```python
from build123d import *

# Parameters (mm, degrees)
BOSS_EXTRUDE1_DEPTH           = 3.175
TAP_DRILL_FOR_8_32_TAP1_D     = 3.4544
TAP_DRILL_FOR_8_32_TAP1_DEPTH = 3.302
TAP_DRILL_FOR_8_32_TAP1_TIP   = 1.037806461
BOSS_EXTRUDE2_DEPTH           = 12.7
F_8_CLEARANCE_HOLE1_D         = 4.9149


with BuildPart() as part:
    # Sketch1 → Boss-Extrude1 (new body)
    with BuildSketch(Plane.XY):
        with BuildLine():
            Line((-9.149583802, 21.93801689), (-26.580783626, -25.95381102))
            Line((-26.580783626, -25.95381102), (20.215712306, -25.95381102))
            Line((20.215712306, -25.95381102), (2.784512482, 21.93801689))
            ThreePointArc((2.784512482, 21.93801689), (-3.18253566, 26.11618898), (-9.149583802, 21.93801689))
        make_face()
    extrude(amount=BOSS_EXTRUDE1_DEPTH)

    # Tap Drill for #8-32 Tap1
    with Locations(Plane(origin=(-3.18253566, 19.76618898, 0), x_dir=(-1, 0, 0), z_dir=(0, 0, -1))):
        with Locations((0, 0)):
            Hole(TAP_DRILL_FOR_8_32_TAP1_D / 2, depth=TAP_DRILL_FOR_8_32_TAP1_DEPTH)
            with Locations((0, 0, -(TAP_DRILL_FOR_8_32_TAP1_DEPTH + TAP_DRILL_FOR_8_32_TAP1_TIP / 2))):  # 118° drill point
                Cone(0, TAP_DRILL_FOR_8_32_TAP1_D / 2, TAP_DRILL_FOR_8_32_TAP1_TIP, mode=Mode.SUBTRACT)

    # Sketch3 → Boss-Extrude2 (add)
    with BuildSketch(Plane(origin=(0, 0, 0), x_dir=(-1, 0, 0), z_dir=(0, 0, -1))):
        Polygon((-19.060106812, -22.77881102), (-20.215712306, -25.95381102), (26.580783626, -25.95381102), (25.425178132, -22.77881102), align=None)
    extrude(amount=BOSS_EXTRUDE2_DEPTH)

    # #8 Clearance Hole1 (through all)
    with Locations(Plane(origin=(-14.303856896, -22.77881102, -6.35), x_dir=(1, 0, 0), z_dir=(0, 1, 0))):
        with Locations((0, 0), (22.242642472, 0)):
            Hole(F_8_CLEARANCE_HOLE1_D / 2)


solid = part.part
```
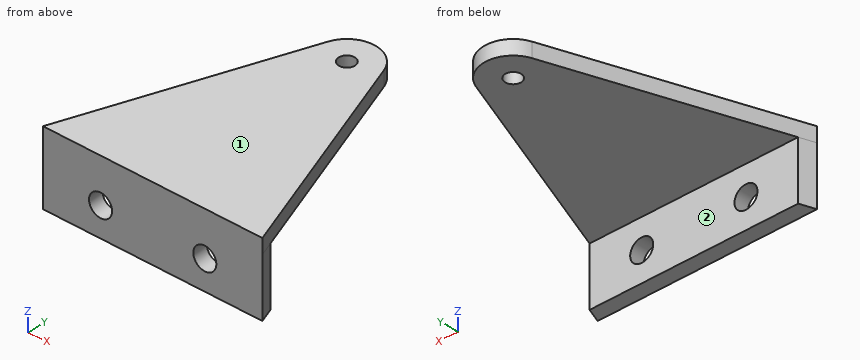
Design review of the part built by this model. Coordinates are the model's own, in mm. Face numbers are marked on the shaded views. A direction names the side the tool comes from. Round coordinates to 2 decimals unless told otherwise and drop trailing zeros. Write each loop counter-clockwise with the first axis right and the second up, starting at its lowest first coordinate (ties: lowest second). Pieces come first, ordered by that corner, then holes.
Item 1: For probe 1 along Z at (x, y) = (-4.5, 10) (3 decimals); probe 2 along Y at (x, z) = (-14, -3.75); probe 3 along X at (y, z) = (-20, 0.5), list the stretches that pass through material, from the lowest coordinate up.
Item 2: We need section B-B on x = 7. Write out the cut boundary in (y, z) (3 decimals).
Item 3: For the marked faces 1 and 2, list the 3-axis set-ups (+Z, -Z, +X, -X, +Y, -Y) from which the entire face can be reached by the end or side of a thin tool; tool diameter is ignored.
Item 4: We need section A-A on z = -6.35. Write out the cut boundary in (x, y), and give its area (3 significant figures).
Item 5: We need section D-D on y = -20.5. Write out the cut boundary in (x, z) (3 decimals).
Item 6: We need section C-C on x = -6. Write out the cut boundary in (y, z) (3 decimals).
Item 7: Clearance check with flat-ended pins moving along their axes: pin 1 Ø1 at (x, z) = (11.5, -4) entering from +Y; pin 2 Ø3 at (x, z) = (7.94, -6.35) entering from +Y; pin 3 Ø22 at (x, y) = (0.5, 9) entering from -Z; pin 4 Ø4 at (y, z) = (14.5, -0.5) entering from +X. State where each tip first meets the part, or that it passes through.
Returned:
1. probe 1: z = 0 to 3.175
1. probe 2: y = -25.95 to -22.78
1. probe 3: x = -24.41 to 18.05
2. outline: (-25.954, -12.7) - (-22.779, -12.7) - (-22.779, -8.621) - (-25.954, -8.621) - close; (-25.954, -4.079) - (-22.779, -4.079) - (-22.779, 0) - (10.356, 0) - (10.356, 3.175) - (-25.954, 3.175) - close
3. face 1: +Z, +X, -X, +Y, -Y
3. face 2: -Z, +X, -X, +Y
4. outline: (-26.58, -25.95) - (-16.76, -25.95) - (-16.76, -22.78) - (-25.43, -22.78) - close; (-11.85, -25.95) - (5.48, -25.95) - (5.48, -22.78) - (-11.85, -22.78) - close; (10.4, -25.95) - (20.22, -25.95) - (19.06, -22.78) - (10.4, -22.78) - close
4. area: 114 mm2
5. outline: (-24.596, 0) - (18.231, 0) - (18.231, 3.175) - (-24.596, 3.175) - close
6. outline: (-25.954, -12.7) - (-22.779, -12.7) - (-22.779, 0) - (25.457, 0) - (25.457, 3.175) - (-25.954, 3.175) - close
7. pin 1: stops at y = -22.78
7. pin 2: passes through
7. pin 3: stops at z = 0
7. pin 4: stops at x = 6.2
